Part print with two shaded views. Sizes in mm from the minimum x, y, z corner. A direction names the side the tool comes from. Round coordinates to 2 decimals unless told otherwise and drop trailing zeros. Order: outer loops, then holes, each group sorted by start corner. A loop starts at its lowest first (then second) coordinate and runs counter-clockwise, first axis right, second up. Notation, with made-up numbers: M 53,45 L 70,45 A21 ccw 70,81 Z; hole C 56.5,-29.5 d5. An arc over 180 degrees is marked long. Put each result on its own line as item: value.
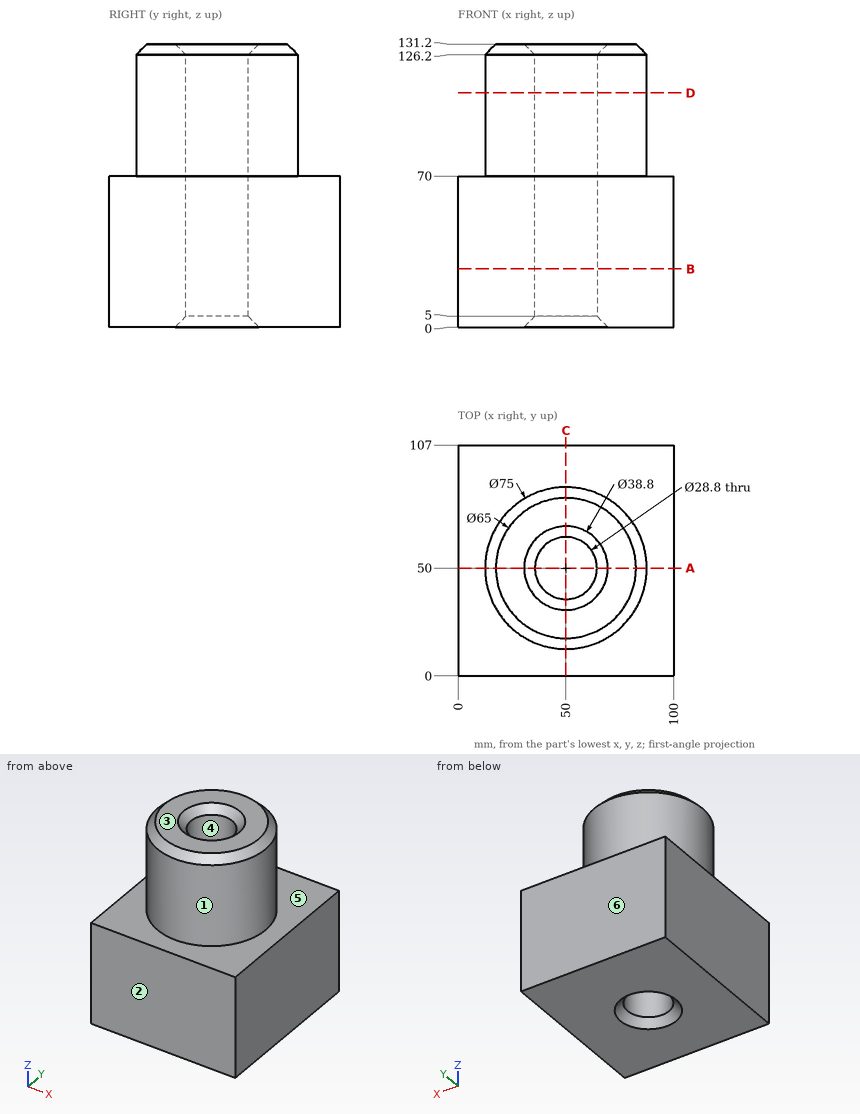
Item 1: Band-saw the part on A-A on y = 50. Give the cut face in (x, z), and give its area (3 significant figures).
Answers below:
outline: M 0,0 L 30.6,0 L 35.6,5 L 35.6,126.2 L 30.6,131.2 L 17.5,131.2 L 12.5,126.2 L 12.5,70 L 0,70 Z; M 64.4,5 L 69.4,0 L 100,0 L 100,70 L 87.5,70 L 87.5,126.2 L 82.5,131.2 L 69.4,131.2 L 64.4,126.2 Z
area: 7,740 mm²
Item 2: Tool access for the marked faces 5 and 6: list every direction of +Z, -Z, +X, -X, +Y, -Y with a clear straight run to the whole face (end or side of a thin tool).
Answers below:
face 5: +Z
face 6: +Z, -Z, +X, -X, +Y
Item 3: Probe line 1 along Y through (x, z) = (50, 54); line 2 along Y through (x, z) = (50, 101); line 3 along Z through (x, y) = (30, 9.5). List the from-to ranges inside material, lowest first. Write a range as [from, to].
Answers below:
line 1: [0, 35.6], [64.4, 107]
line 2: [12.5, 35.6], [64.4, 87.5]
line 3: [0, 70]
Item 4: Mould opens along Y. For the marked faces 1, 2, 3 and 4 say: pulls with the +Y half, pulls with the -Y half, needs draft (parallel to the pull), parting line crosses it, or undercut.
Answers below:
face 1: parting line crosses it
face 2: pulls with the -Y half
face 3: needs draft
face 4: undercut
Item 5: Band-saw the part on B-B on z = 27. Give the cut face in (x, y), and give its area (3 significant figures).
Answers below:
outline: M 0,0 L 100,0 L 100,107 L 0,107 Z; hole C 50,50 d28.8
area: 10,000 mm²
Item 6: Pin check, flat tips, straight feed: P1, Ø8, axis at x = 69, z = 94, coming from the +Y side; P2, Ø4, axis at x = 22, z = 96, coming from the +Y side; P3, Ø1.5, axis at y = 66.5, z = 91, coming from the -X side. Stop position of each tip, or through.
Answers below:
P1: y = 84.37
P2: y = 77.02
P3: x = 15.97
Item 7: Band-saw the part on D-D on z = 108.5. Give the cut face in (x, y).
Answers below:
outline: C 50,50 d75; hole C 50,50 d28.8
Item 8: Band-saw the part on C-C on x = 50. Give the cut face in (y, z), and give its area (3 significant figures).
Answers below:
outline: M 0,0 L 30.6,0 L 35.6,5 L 35.6,126.2 L 30.6,131.2 L 17.5,131.2 L 12.5,126.2 L 12.5,70 L 0,70 Z; M 64.4,5 L 69.4,0 L 107,0 L 107,70 L 87.5,70 L 87.5,126.2 L 82.5,131.2 L 69.4,131.2 L 64.4,126.2 Z
area: 8,230 mm²
